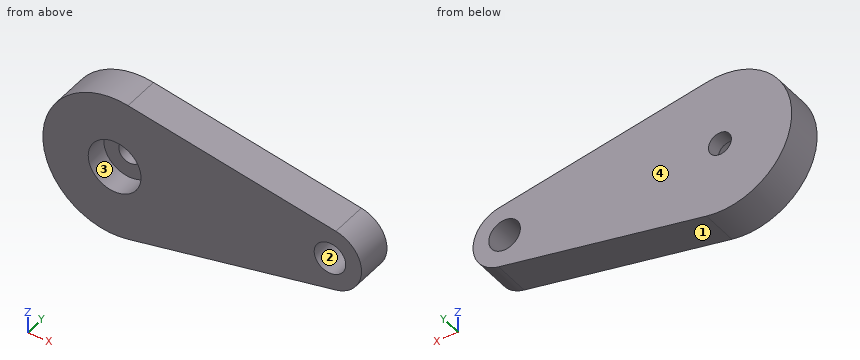
Autodesk Inventor part; units mm, degrees
ref_plane "YZ Plane" through (0, 0, 0) normal (1, 0, 0) x (0, 1, 0)
ref_plane "XZ Plane" through (0, 0, 0) normal (0, 1, 0) x (-1, 0, 0)
ref_plane "XY Plane" through (0, 0, 0) normal (0, 0, 1) x (1, 0, 0)
sketch "Sketch1" plane through (0, 0, 0) normal (0, 1, 0) x (-1, 0, 0)
  circle A0 centre (0, 0) radius 2.3368
  arc A1 (-1.1853, -6.2384) -> (-1.1853, 6.2384) centre (0, 0) ccw
  arc A2 (-19.5715, 2.7449) -> (-19.5715, -2.7449) centre (-19.05, 0) ccw
  line L0 (-1.1853, -6.2384) -> (-19.5715, -2.7449)
  line L1 (-19.5715, 2.7449) -> (-1.1853, 6.2384)
  circle A3 centre (-19.05, 0) radius 1.397
  arc A4 (-2.3333, -0.127) -> (-2.3333, 0.127) centre (-2.3368, 0) ccw
  arc A5 (-2.256, -0.6093) -> (-2.3088, -0.361) centre (-2.2857, -0.4858) ccw
  arc A6 (-2.08, -1.065) -> (-2.1833, -0.8331) centre (-2.1348, -0.9505) ccw
  arc A7 (-1.8131, -1.4742) -> (-1.9623, -1.2688) centre (-1.8905, -1.3735) ccw
  arc A8 (-1.467, -1.819) -> (-1.6557, -1.6491) centre (-1.5636, -1.7366) ccw
  arc A9 (-1.0567, -2.0842) -> (-1.2766, -1.9573) centre (-1.1684, -2.0237) ccw
  arc A10 (-0.6003, -2.2584) -> (-0.8418, -2.1799) centre (-0.7221, -2.2224) ccw
  arc A11 (-0.1176, -2.3338) -> (-0.3702, -2.3073) centre (-0.2443, -2.324) ccw
  arc A12 (0.3702, -2.3073) -> (0.1176, -2.3338) centre (0.2443, -2.324) ccw
  arc A13 (0.8418, -2.1799) -> (0.6003, -2.2584) centre (0.7221, -2.2224) ccw
  arc A14 (1.2766, -1.9573) -> (1.0567, -2.0842) centre (1.1684, -2.0237) ccw
  arc A15 (1.6557, -1.6491) -> (1.467, -1.819) centre (1.5636, -1.7366) ccw
  arc A16 (1.9623, -1.2688) -> (1.8131, -1.4742) centre (1.8905, -1.3735) ccw
  arc A17 (2.1833, -0.8331) -> (2.08, -1.065) centre (2.1348, -0.9505) ccw
  arc A18 (2.3088, -0.361) -> (2.256, -0.6093) centre (2.2857, -0.4858) ccw
  arc A19 (2.3333, 0.127) -> (2.3333, -0.127) centre (2.3368, 0) ccw
  arc A20 (2.256, 0.6093) -> (2.3088, 0.361) centre (2.2857, 0.4858) ccw
  arc A21 (2.08, 1.065) -> (2.1833, 0.8331) centre (2.1348, 0.9505) ccw
  arc A22 (1.8131, 1.4742) -> (1.9623, 1.2688) centre (1.8905, 1.3735) ccw
  arc A23 (1.467, 1.819) -> (1.6557, 1.6491) centre (1.5636, 1.7366) ccw
  arc A24 (1.0567, 2.0842) -> (1.2766, 1.9573) centre (1.1684, 2.0237) ccw
  arc A25 (0.6003, 2.2584) -> (0.8418, 2.1799) centre (0.7221, 2.2224) ccw
  arc A26 (0.1176, 2.3338) -> (0.3702, 2.3073) centre (0.2443, 2.324) ccw
  arc A27 (-0.3702, 2.3073) -> (-0.1176, 2.3338) centre (-0.2443, 2.324) ccw
  arc A28 (-0.8418, 2.1799) -> (-0.6003, 2.2584) centre (-0.7221, 2.2224) ccw
  arc A29 (-1.2766, 1.9573) -> (-1.0567, 2.0842) centre (-1.1684, 2.0237) ccw
  arc A30 (-1.6557, 1.6491) -> (-1.467, 1.819) centre (-1.5636, 1.7366) ccw
  arc A31 (-1.9623, 1.2688) -> (-1.8131, 1.4742) centre (-1.8905, 1.3735) ccw
  arc A32 (-2.1833, 0.8331) -> (-2.08, 1.065) centre (-2.1348, 0.9505) ccw
  arc A33 (-2.3088, 0.361) -> (-2.256, 0.6093) centre (-2.2857, 0.4858) ccw
  point P0 (-2.256, -0.6093)
  point P1 (-2.3088, -0.361)
  point P2 (-2.1833, -0.8331)
  point P3 (-1.8131, -1.4742)
  point P4 (-1.6557, -1.6491)
  point P5 (-1.0567, -2.0842)
  point P6 (-0.8418, -2.1799)
  point P7 (-0.1176, -2.3338)
  point P8 (-0.3702, -2.3073)
  point P9 (0.1176, -2.3338)
  point P10 (0.8418, -2.1799)
  point P11 (0.6003, -2.2584)
  point P12 (1.8131, -1.4742)
  point P13 (2.08, -1.065)
  point P14 (2.3088, -0.361)
  point P15 (2.256, -0.6093)
  point P16 (2.256, 0.6093)
  point P17 (2.3088, 0.361)
  point P18 (2.1833, 0.8331)
  point P19 (1.9623, 1.2688)
  point P20 (1.6557, 1.6491)
  point P21 (1.0567, 2.0842)
  point P22 (1.2766, 1.9573)
  point P23 (0.6003, 2.2584)
  point P24 (0.8418, 2.1799)
  point P25 (0.1176, 2.3338)
  point P26 (0.3702, 2.3073)
  point P27 (-0.1176, 2.3338)
  point P28 (-0.8418, 2.1799)
  point P29 (-0.6003, 2.2584)
  point P30 (-1.2766, 1.9573)
  point P31 (-1.0567, 2.0842)
  point P32 (-1.8131, 1.4742)
  point P33 (-2.08, 1.065)
  point P34 (-2.3088, 0.361)
  point P35 (-2.256, 0.6093)
  dimension "d0" = 4.6736
  dimension "d1" = 12.7
  dimension "d2" = 19.05
  dimension "d3" = 5.588
  dimension "d4" = 2.794
  dimension "d10" = 0.254
  dimension "d13" = 360
extrude "Extrusion1" add sketch "Sketch1" along normal blind 2.032
sketch "Sketch2" plane through (0, 2.032, 0) normal (0, 1, 0) x (1, 0, 0)
  line L0 (19.5715, 2.7449) -> (1.1853, 6.2384)
  arc A0 (1.1853, 6.2384) -> (1.1853, -6.2384) centre (0, 0) ccw
  line L1 (1.1853, -6.2384) -> (19.5715, -2.7449)
  arc A1 (19.5715, -2.7449) -> (19.5715, 2.7449) centre (19.05, 0) ccw
  circle A2 centre (0, 0) radius 2.3368
  circle A3 centre (19.05, 0) radius 1.397
  circle A4 centre (0, 0) radius 1.016
  dimension "d7" = 2.032
extrude "Extrusion2" add sketch "Sketch2" along normal blind 1.27 contours A1 L1 A0 L0 | A2
properties part number "Servo Spinner"
The model under review builds one solid part; all positions refer to its coordinate system, in mm. Face numbers are marked on the shaded views. Give positions to 0.01 mm unless a question says otherwise; leave off trailing zeros. Order: outer loops, then holes, each group sorted by start corner. A loop starts at its lowest first (then second) coordinate and runs counter-clockwise, first axis right, second up. Notation, with made-up numbers: M 4.25,18.25 L 62.25,18.25 A16 cw 62.25,38.25 Z; hole C -37,75.5 d10. An arc over 180 degrees is marked long. Use one line per item in the form item = value. Start each with the question number.
Item 1: We need section D-D on y = 2.8. Give the boundary of the cut face in (x, z), plus the area to 3 significant figures.
Item 2: The part is to be moulded in two halves that separate along X. For the marked faces 1, 2, 3 and 4, say which applies: pulls with the +X half, pulls with the -X half, needs draft (parallel to the pull), parting line crosses it, or undercut.
Item 3: We need section C-C on z = -1.75. Give the boundary of the cut face in (x, y), plus the area to 3 significant figures.
Item 4: Insertion check: pin 1 Ø1.7 at (x, z) = (19.05, 0) entering from +Y. The pin has a flat end and moves straight along its axis. Give the tip position at first contact, or say it passes through.
Item 5: We need section A-A on x = 0. Give the boundary of the cut face in (y, z), plus the area to 3 significant figures.
Item 6: To check wall thickness, follow line 1 along X through (y, z) = (2.45, 0); line 2 along Z through (x, y) = (0, 3); line 3 along X through (y, z) = (0.35, -0.5). State the ranges of each line that lie inside material, in increasing order. Write a range as from..to.
Item 7: We need section B-B on y = 0.9. Give the boundary of the cut face in (x, z), plus the area to 3 significant figures.
Completed:
q1.outline = M 1.19,-6.24 L 19.57,-2.74 A2.79 ccw 19.57,2.74 L 1.19,6.24 A6.35 ccw long Z; hole C 0,0 d2.03; hole C 19.05,0 d2.79
q1.area = 243 mm²
q2.face_1 = pulls with the +X half
q2.face_2 = undercut
q2.face_3 = undercut
q2.face_4 = needs draft
q3.outline = M -6.1,0 L -1.55,0 L -1.55,2.03 L 1.55,2.03 L 1.55,0 L 21.23,0 L 21.23,3.3 L -6.1,3.3 Z
q3.area = 84.0 mm²
q4.pin_1 = through
q5.outline = M 0,-6.35 L 3.3,-6.35 L 3.3,-1.02 L 2.03,-1.02 L 2.03,-2.34 L 0,-2.34 Z; M 0,2.34 L 2.03,2.34 L 2.03,1.02 L 3.3,1.02 L 3.3,6.35 L 0,6.35 Z
q5.area = 29.9 mm²
q6.line_1 = -6.35..-1.02, 1.02..17.65, 20.45..21.84
q6.line_2 = -6.35..-1.02, 1.02..6.35
q6.line_3 = -6.33..-2.28, 2.28..17.75, 20.35..21.8
q7.outline = M 1.19,-6.24 L 19.57,-2.74 A2.79 ccw 19.57,2.74 L 1.19,6.24 A6.35 ccw long Z; hole C 0,0 d4.67; hole C 19.05,0 d2.79
q7.area = 230 mm²
